```python
from build123d import *

# Parameters (mm, degrees)
SKETCH1_W           = 73
SKETCH1_H           = 36
BOSS_EXTRUDE1_DEPTH = 2
SKETCH2_W           = 1.5
SKETCH2_H           = 19
BOSS_EXTRUDE2_DEPTH = 6
SKETCH3_W           = 25.4
SKETCH3_H           = 27.4
SKETCH3_W_2         = 22.4
SKETCH3_H_2         = 24.4
BOSS_EXTRUDE3_DEPTH = 10
SKETCH4_W           = 22.4
SKETCH4_H           = 19
CUT_EXTRUDE1_DEPTH  = 42.907636536
SKETCH5_W           = 22.4
SKETCH5_H           = 1.5
BOSS_EXTRUDE4_DEPTH = 6
SKETCH6_R           = 1.5
CUT_EXTRUDE2_DEPTH  = 43.429353047
SKETCH7_W           = 1.5
SKETCH7_H           = 19
BOSS_EXTRUDE5_DEPTH = 2.5
SKETCH8_R           = 1.7
CUT_EXTRUDE3_DEPTH  = 54.335166635


with BuildPart() as part:
    # Sketch1 → Boss-Extrude1 (new body)
    with BuildSketch(Plane(origin=(0, 0, 0), x_dir=(1, 0, 0), z_dir=(0, 1, 0))):
        Rectangle(SKETCH1_W, SKETCH1_H)
    extrude(amount=BOSS_EXTRUDE1_DEPTH)

    # Sketch2 → Boss-Extrude2 (add)
    with BuildSketch(Plane(origin=(0, 2, 0), x_dir=(1, 0, 0), z_dir=(0, 1, 0))):
        with Locations((-35.75, 0)):
            Rectangle(SKETCH2_W, SKETCH2_H)
        with Locations((35.75, 0)):
            Rectangle(SKETCH2_W, SKETCH2_H)
    extrude(amount=BOSS_EXTRUDE2_DEPTH)

    # Sketch3 → Boss-Extrude3 (add)
    with BuildSketch(Plane.XZ):
        Rectangle(SKETCH3_W, SKETCH3_H)
        Rectangle(SKETCH3_W_2, SKETCH3_H_2, mode=Mode.SUBTRACT)
    extrude(amount=BOSS_EXTRUDE3_DEPTH)

    # Sketch4 → Cut-Extrude1 (cut, through all)
    with BuildSketch(Plane.XZ):
        Rectangle(SKETCH4_W, SKETCH4_H)
    extrude(amount=-CUT_EXTRUDE1_DEPTH, mode=Mode.SUBTRACT)

    # Sketch5 → Boss-Extrude4 (add)
    with BuildSketch(Plane(origin=(0, 2, 0), x_dir=(1, 0, 0), z_dir=(0, 1, 0))):
        with Locations((0, 10.25)):
            Rectangle(SKETCH5_W, SKETCH5_H)
        with Locations((0, -10.25)):
            Rectangle(SKETCH5_W, SKETCH5_H)
    extrude(amount=BOSS_EXTRUDE4_DEPTH)

    # Sketch6 → Cut-Extrude2 (cut, through all)
    with BuildSketch(Plane(origin=(0, 2, 0), x_dir=(1, 0, 0), z_dir=(0, 1, 0))):
        with Locations(Location((-26.5, 9.5, 0), (0, 0, 270))):
            Circle(SKETCH6_R)
        with Locations(Location((-26.5, -9.5, 0), (0, 0, 270))):
            Circle(SKETCH6_R)
        with Locations(Location((26.5, 9.5, 0), (0, 0, 270))):
            Circle(SKETCH6_R)
        with Locations(Location((26.5, -9.5, 0), (0, 0, 270))):
            Circle(SKETCH6_R)
    extrude(amount=-CUT_EXTRUDE2_DEPTH, mode=Mode.SUBTRACT)

    # Sketch7 → Boss-Extrude5 (add)
    with BuildSketch(Plane(origin=(0, 2, 0), x_dir=(1, 0, 0), z_dir=(0, 1, 0))):
        with Locations((-31.5, 0)):
            Rectangle(SKETCH7_W, SKETCH7_H)
        with Locations((31.5, 0)):
            Rectangle(SKETCH7_W, SKETCH7_H)
    extrude(amount=BOSS_EXTRUDE5_DEPTH)

    # Sketch8 → Cut-Extrude3 (cut, through all)
    with BuildSketch(Plane(origin=(12.7, 0, 0), x_dir=(0, 0, -1), z_dir=(1, 0, 0))):
        with Locations((-8, -6.5)):
            Circle(SKETCH8_R)
        with Locations((8, -6.5)):
            Circle(SKETCH8_R)
    extrude(amount=-CUT_EXTRUDE3_DEPTH, mode=Mode.SUBTRACT)


solid = part.part
```
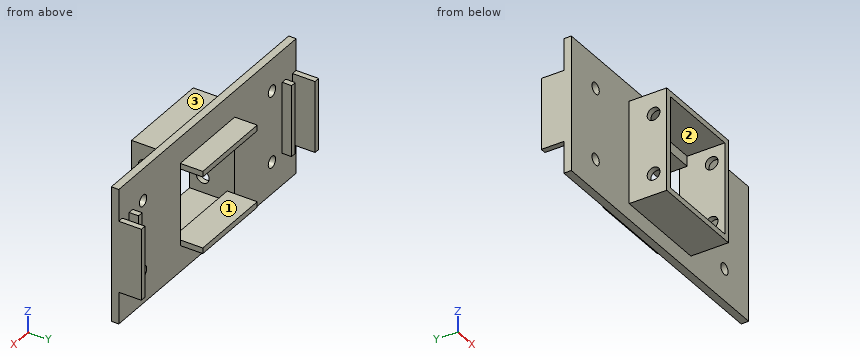
Geometry: final body of the model. Coordinates: model frame, mm. Face numbers are marked on the shaded views. A direction names the side the tool comes from. Round coordinates to 2 decimals unless told otherwise and drop trailing zeros. Loops run counter-clockwise (first coordinate to the right, second up) from the corner with the lowest first, then second, coordinate; pieces in that order, holes last.
Item 1: Section B-B, the plane x = -12. Output: boundary loops of the cut face in (y, z).
Checked values:
outline: (-10, -13.7) - (0, -13.7) - (0, -18) - (2, -18) - (2, 18) - (0, 18) - (0, 13.7) - (-10, 13.7) - close; hole circle Ø3.4 at (-6.5, -8); hole circle Ø3.4 at (-6.5, 8)
Item 2: Reachability of the marked faces 1, 2 and 3 from +Z, -Z, +X, -X, +Y, -Y: full face, straight path, thin tool, end or side. Return the list, or none.
Checked values:
face 1: +Y, -Y
face 2: -Y
face 3: +Z, +X, -X, -Y
Item 3: Contact query for flat-ended pins moving along their axis: P1, Ø1.6, axis at x = 35.5, y = 5, coming from the +Z side; P2, Ø3, axis at x = 4.5, y = -2.5, coming from the +Z side; P3, Ø4, axis at x = 14.5, z = -13.5, coming from the +Y side; P4, Ø8, axis at x = -8, y = 3, coming from the -Z side. Output: stop coordinate, or through.
Checked values:
P1: stops at z = 9.5
P2: stops at z = 13.7
P3: stops at y = 2
P4: stops at z = -18
Item 4: Line query: L1, parallel to X at y = 3.25, z = -7; L2, parallel to X at y = -0.5, z = 8.5; L3, parallel to Y at x = 12.25, z = 8. Output: solid intervals per line, ascending.
Checked values:
L1: x = -36.5 to -35, -32.25 to -30.75, 30.75 to 32.25, 35 to 36.5
L2: x = -12.7 to -11.2, 11.2 to 12.7
L3: y = -10 to -8.2, -4.8 to 2
Item 5: Section D-D, the plane y = 3. Output: boundary loops of the cut face in (x, z), plus the area to 3 significant figures.
Checked values:
outline: (-36.5, -9.5) - (-35, -9.5) - (-35, 9.5) - (-36.5, 9.5) - close; (-32.25, -9.5) - (-30.75, -9.5) - (-30.75, 9.5) - (-32.25, 9.5) - close; (-11.2, -11) - (11.2, -11) - (11.2, -9.5) - (-11.2, -9.5) - close; (-11.2, 9.5) - (11.2, 9.5) - (11.2, 11) - (-11.2, 11) - close; (30.75, -9.5) - (32.25, -9.5) - (32.25, 9.5) - (30.75, 9.5) - close; (35, -9.5) - (36.5, -9.5) - (36.5, 9.5) - (35, 9.5) - close
area: 181 mm2
Item 6: Section C-C, the plane x = -26.5. Output: boundary loops of the cut face in (y, z), plus the area to 3 significant figures.
Checked values:
outline: (0, -18) - (2, -18) - (2, -11) - (0, -11) - close; (0, -8) - (2, -8) - (2, 8) - (0, 8) - close; (0, 11) - (2, 11) - (2, 18) - (0, 18) - close
area: 60.0 mm2
Item 7: Section A-A, the plane y = 6.75. Output: boundary loops of the cut face in (x, z), plus the area to 3 significant figures.
Checked values:
outline: (-36.5, -9.5) - (-35, -9.5) - (-35, 9.5) - (-36.5, 9.5) - close; (-11.2, -11) - (11.2, -11) - (11.2, -9.5) - (-11.2, -9.5) - close; (-11.2, 9.5) - (11.2, 9.5) - (11.2, 11) - (-11.2, 11) - close; (35, -9.5) - (36.5, -9.5) - (36.5, 9.5) - (35, 9.5) - close
area: 124 mm2
